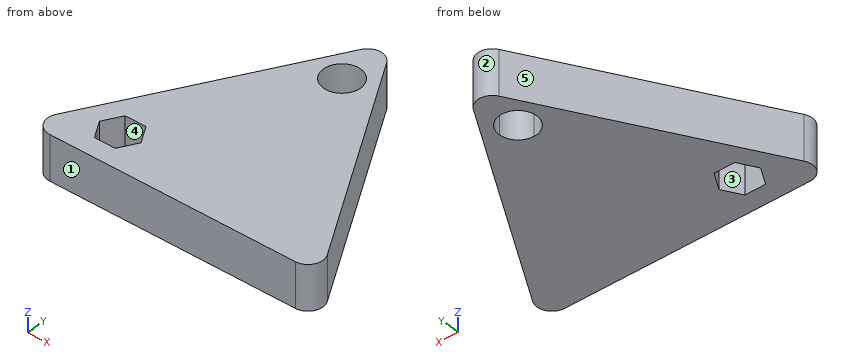
```python
from build123d import *

# Parameters (mm, degrees)
F1_DEPTH = 15
F2_R     = 5


with BuildPart() as f1:
    # F0 (on Top) → F1 (new body)
    with BuildSketch(Plane.XY):
        Polygon((50, -46.6025403784), (0, 40), (-50, -46.6025403784), align=None)
        Polygon((-31.8494454538, -40.1648577189), (-33.599485728, -37.1336990487), (-35.3495260022, -34.1025403784), (-31.8494454538, -28.040223038), (-24.849284357, -28.040223038), (-21.3492038085, -34.1025403784), (-24.849284357, -40.1648577189), align=None, mode=Mode.SUBTRACT)
        with BuildLine():
            ThreePointArc((0, 13.75), (-4.4194173824, 24.4194173824), (6.25, 20))
            ThreePointArc((6.25, 20), (4.4194173824, 15.5805826176), (0, 13.75))
        make_face(mode=Mode.SUBTRACT)
    extrude(amount=F1_DEPTH)

    # F2
    f2_edges = [f1.edges().sort_by_distance(p)[0] for p in [
        (-50, -46.60254, 7.5),
        (50, -46.60254, 7.5),
        (0, 40, 7.5),
    ]]
    fillet(f2_edges, radius=F2_R)


solid = f1.part
```
Here's how the part is built. I have some questions about the finished solid (model axes, mm). Face numbers are marked on the shaded views. A direction names the side the tool comes from. Give positions to 0.01 mm unless a question says otherwise; leave off trailing zeros. Order: outer loops, then holes, each group sorted by start corner. A loop starts at its lowest first (then second) coordinate and runs counter-clockwise, first axis right, second up. Notation, with made-up numbers: (16, -21) - (33, -21) arc R22 ccw to (33, -3) - close; hole circle Ø2 at (27, 10). An arc over 180 degrees is marked (long way). Answer as a JSON object with one key per item and string values. Group by question number.
Item 1: If we section it at B-B on y = -32: Please give me the cut outline in (x, z).
Item 2: Please list where these lines run through material, in increasing order: probe 1 along Y at (x, z) = (2.5, 4); probe 2 along X at (y, z) = (20, 9.25); probe 3 along Y at (x, z) = (5, 10).
Item 3: For P1, Ø8, axis at y = 23, z = 11, coming from the -X side; P2, Ø1, axis at y = 21, z = 4, coming from the +X side; P3, Ø3.5, axis at x = -29, z = 5, coming from the +Y side, each with a flat end and sliding along its axis, tell me the tip position at first contact or that it passes through.
Item 4: If we section it at A-A on z = 5: Please give me the cut outline in (x, y), and give its area (3 significant figures).
Item 5: Which directions (+Z, -Z, +X, -X, +Y, -Y) give clear straight access to the entire face, cutting with the end or side of a thin tool? Please do the marked faces 4 and 5.
Item 6: If we section it at D-D on x = 27: Please give me the cut outline in (y, z).
Item 7: If we mould it in two halves opening along X, with no side actions, what happens to the marked faces 1, 2 and 3? For each: pulls with the +X half, pulls with the -X half, needs draft (parallel to the pull), parting line crosses it, or undercut.
Item 8: If we section it at C-C on y = -11: Please give me the cut outline in (x, z).
Result set:
{
 "1": {"outline": "(-41.57, 0) - (-34.14, 0) - (-34.14, 15) - (-41.57, 15) - close; (-22.56, 0) - (41.57, 0) - (41.57, 15) - (-22.56, 15) - close"},
 "2": {"probe 1": "-46.6 to 14.27, 25.73 to 34.33", "probe 2": "-11.55 to -6.25, 6.25 to 11.55", "probe 3": "-46.6 to 16.25, 23.75 to 31.34"},
 "3": {"P1": "x = -12.12", "P2": "x = 11.26", "P3": "y = -7.2"},
 "4": {"outline": "(-45.67, -39.1) arc R5 ccw to (-41.34, -46.6) - (41.34, -46.6) arc R5 ccw to (45.67, -39.1) - (4.33, 32.5) arc R5 ccw to (-4.33, 32.5) - close; hole (-35.35, -34.1) - (-31.85, -40.16) - (-24.85, -40.16) - (-21.35, -34.1) - (-24.85, -28.04) - (-31.85, -28.04) - close; hole circle Ø12.5 at (0, 20)", "area": "4,030 mm²"},
 "5": {"face 4": "+Z, -Z", "face 5": "+Z, -Z, -X, +Y"},
 "6": {"outline": "(-46.6, 0) - (-6.77, 0) - (-6.77, 15) - (-46.6, 15) - close"},
 "7": {"face 1": "needs draft", "face 2": "parting line crosses it", "face 3": "undercut"},
 "8": {"outline": "(-29.44, 0) - (29.44, 0) - (29.44, 15) - (-29.44, 15) - close"}
}
